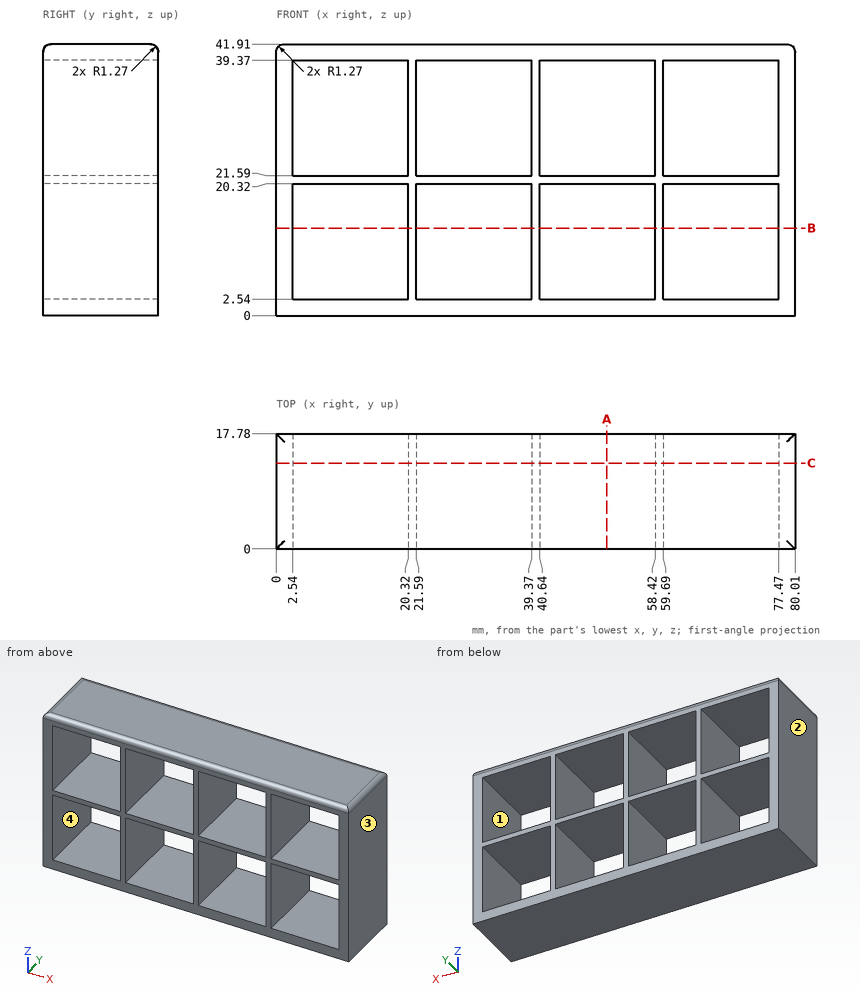
Check sheet for the drawn part. Datum: minimum x, y, z corner. Units: mm. A direction names the side the tool comes from. Coordinates: 2 decimals unless noted, no trailing zeros. Write each loop counter-clockwise with the first axis right and the second up, starting at its lowest first coordinate (ties: lowest second). Pieces come first, ordered by that corner, then holes. Notation, with made-up numbers: M -17.75,68 L -5.75,68 A5 ccw -5.75,76 Z; hole C 11,40.25 d6. An arc over 180 degrees is marked long. One line per item, written item: value.
Item 1: Mould release check, pull along Z, two halves, no side actions. Record for the marked faces 1 and 2: pulls with the +Z half, pulls with the -Z half, needs draft (parallel to the pull), parting line crosses it, or undercut.
Check sheet entries:
face 1: undercut
face 2: needs draft
Item 2: Section check C-C, the plane y = 13.25. State how many separate pieces and enclosed holes the cut face has, plus the area to 4 significant figures.
Check sheet entries:
separate pieces: 1
enclosed holes: 8
area: 823.5 mm^2
Item 3: Section check A-A, the plane x = 51. Record the boundary of the cut face in (y, z).
Check sheet entries:
outline: M 0,0 L 17.78,0 L 17.78,2.54 L 0,2.54 Z; M 0,20.32 L 17.78,20.32 L 17.78,21.59 L 0,21.59 Z; M 0,39.37 L 17.78,39.37 L 17.78,40.64 A1.27 ccw 16.51,41.91 L 1.27,41.91 A1.27 ccw 0,40.64 Z
Item 4: Scan lines: line 1 along X through (y, z) = (4, 34); line 2 along Z through (x, y) = (50, 5). Record each from-to range of solid material in increasing order.
Check sheet entries:
line 1: x = 0 to 2.54, 20.32 to 21.59, 39.37 to 40.64, 58.42 to 59.69, 77.47 to 80.01
line 2: z = 0 to 2.54, 20.32 to 21.59, 39.37 to 41.91
Item 5: Gauge pin test, flat ends, axial feed: pin 1 Ø12 at (x, z) = (51, 27.5) entering from +Y; pin 2 Ø6 at (x, z) = (66, 16) entering from -Y. Record the tip position at first contact, or that the pin passes through.
Check sheet entries:
pin 1: stops at y = 17.78
pin 2: passes through
Item 6: Access from +Z, -Z, +X, -X, +Y, -Y to the whole of each face (thin tool, end or side, straight path). Record for the marked faces 3 and 4.
Check sheet entries:
face 3: +Z, -Z, +X, +Y, -Y
face 4: +Y, -Y
Item 7: Section check B-B, the plane z = 13.5. Record the boundary of the cut face in (x, y).
Check sheet entries:
outline: M 0,0 L 2.54,0 L 2.54,17.78 L 0,17.78 Z; M 20.32,0 L 21.59,0 L 21.59,17.78 L 20.32,17.78 Z; M 39.37,0 L 40.64,0 L 40.64,17.78 L 39.37,17.78 Z; M 58.42,0 L 59.69,0 L 59.69,17.78 L 58.42,17.78 Z; M 77.47,0 L 80.01,0 L 80.01,17.78 L 77.47,17.78 Z
